```python
from build123d import *

# Parameters (mm, degrees)
F0_R     = 4
F1_DEPTH = 10
F2_R     = 3
F3_DEPTH = 10.001
F2_R_2   = 5.25
F4_DEPTH = 5


with BuildPart() as f1:
    # F0 (on Top) → F1 (new body, symmetric)
    with BuildSketch(Plane.XY):
        Polygon((-9, 5), (-30, 5), (-30, -5), (30, -5), (30, 5), (9, 5), align=None)
        with BuildLine():
            Line((-9, 25), (-9, 5))
            Line((-9, 5), (9, 5))
            Line((9, 5), (9, 25))
            ThreePointArc((9, 25), (0, 34), (-9, 25))
        make_face()
        with Locations((0, 25)):
            Circle(F0_R, mode=Mode.SUBTRACT)
    extrude(amount=F1_DEPTH, both=True)

    # F2 (on face) → F3 (cut, through all)
    with BuildSketch(Plane(origin=(0, 5, 0), x_dir=(-1, 0, 0), z_dir=(0, 1, 0))):
        with Locations((20, 0)):
            Circle(F2_R)
        with Locations((-20, 0)):
            Circle(F2_R)
    extrude(amount=-F3_DEPTH, mode=Mode.SUBTRACT)

    # F2 (on face) → F4 (cut)
    with BuildSketch(Plane(origin=(0, 5, 0), x_dir=(-1, 0, 0), z_dir=(0, 1, 0))):
        with Locations((20, 0)):
            Circle(F2_R_2)
        with Locations((20, 0)):
            Circle(F2_R, mode=Mode.SUBTRACT)
        with Locations((-20, 0)):
            Circle(F2_R_2)
        with Locations((-20, 0)):
            Circle(F2_R, mode=Mode.SUBTRACT)
    extrude(amount=-F4_DEPTH, mode=Mode.SUBTRACT)


solid = f1.part
```
Verification items for the finished model (mm, model axes). A direction names the side the tool comes from. Give positions to 0.01 mm unless a question says otherwise; leave off trailing zeros. Loops run counter-clockwise (first coordinate to the right, second up) from the corner with the lowest first, then second, coordinate; pieces in that order, holes last. Notation, with made-up numbers: M 4.5,-32.5 L 37.5,-32.5 A29 cw 37.5,-12.5 Z; hole C -33.5,37.5 d1. An arc over 180 degrees is marked long. One line per question, with ' | ' between items.
Item 1: Tool access check on faces 5 (the face through (-9, 15, 0)), 6 (the face through (25.245, 2.535, 0.231)), 7 (the face through (30, 0, 0)), 8 (the face through (17, 5, 5)), 9 (the face through (-0.521, 28.966, -0.14)). Record the directions out of +Z, -Z, +X, -X, +Y, -Y that give a thin tool (end or side, any length) a straight path to the whole face; none if there is none.
Completed:
face 5: +Z, -Z, -X, +Y | face 6: +Y | face 7: +Z, -Z, +X, +Y, -Y | face 8: +Z, -Z, +X, +Y | face 9: +Z, -Z
Item 2: Section check C-C, the plane y = 1. Record the cut outline in (x, z), plus the area to 3 significant figures.
Completed:
outline: M -30,-10 L 30,-10 L 30,10 L -30,10 Z; hole C -20,0 d10.5; hole C 20,0 d10.5 | area: 1,030 mm^2
Item 3: Draft check along Z on faces 1 (the face through (-14.755, 2.535, 0.231)), 2 (the face through (0, -5, 0)), 3 (the face through (0, 6, 10)), 4 (the face through (0, 6, -10)). Enter one of: +Z half, -Z half, draft (parallel to the pull), parting line (faces both ways), or undercut.
Completed:
face 1: undercut | face 2: draft | face 3: +Z half | face 4: -Z half
Item 4: Section check D-D, the plane z = 6. Record the cut outline in (x, y), plus the area to 3 significant figures.
Completed:
outline: M -30,-5 L 30,-5 L 30,5 L 9,5 L 9,25 A9 ccw -9,25 L -9,5 L -30,5 Z; hole C 0,25 d8 | area: 1,040 mm^2
Item 5: Section check B-B, the plane x = 0. Record the cut outline in (y, z).
Completed:
outline: M -5,-10 L 21,-10 L 21,10 L -5,10 Z; M 29,-10 L 34,-10 L 34,10 L 29,10 Z
Item 6: Thickness scan on line 1 (Z direction, x = 20, y = 1.55); line 2 (X direction, y = 6, z = -6.5); line 3 (Y direction, x = -13, z = 0.75). Record the ranges inside material, lowest first. Write a range as [from, to].
Completed:
line 1: z = [-10, -5.25], [5.25, 10] | line 2: x = [-9, 9] | line 3: y = [-5, 5]
Item 7: Depth check by flat-ended pin: P1, Ø8, axis at y = 20.5, z = 2.5, coming from the -X side; P2, Ø9.5, axis at x = -20, z = 0, coming from the +Y side; P3, Ø6, axis at y = 17, z = -5.5, coming from the +X side. Enter the tip coordinate at first touch or a pass-through.
Completed:
P1: stops at x = -9 | P2: stops at y = 0 | P3: stops at x = 9
Item 8: Section check A-A, the plane z = 0. Record the cut outline in (x, y).
Completed:
outline: M -30,-5 L -23,-5 L -23,0 L -25.25,0 L -25.25,5 L -30,5 Z; M -17,-5 L 17,-5 L 17,0 L 14.75,0 L 14.75,5 L 9,5 L 9,25 A9 ccw -9,25 L -9,5 L -14.75,5 L -14.75,0 L -17,0 Z; M 23,-5 L 30,-5 L 30,5 L 25.25,5 L 25.25,0 L 23,0 Z; hole C 0,25 d8
